Solid Edge part; units mm, degrees
sketch "Sketch1" plane through (0, 0, 0) normal (0, 0, 1) x (1, 0, 0)
  circle A0 centre (0, 0) radius 5
extrude "Protrusion1" add sketch "Sketch1" along normal blind 1.5
sketch "Sketch2" plane through (0, 0, 0) normal (0, 0, 1) x (1, 0, 0)
  line L0 (-1, 4) -> (-1, -4)
  line L1 (-1, -4) -> (1, -4)
  line L2 (1, -4) -> (1, 4)
  line L3 (1, 4) -> (-1, 4)
extrude "Protrusão_Extrudada_2" add sketch "Sketch2" along normal blind 2.3
sketch "Sketch3" plane through (0, 0, 0) normal (0, 0, 1) x (1, 0, 0)
  line L0 (-4, -1) -> (4, -1)
  line L1 (4, -1) -> (4, 1)
  line L2 (4, 1) -> (-4, 1)
  line L3 (-4, 1) -> (-4, -1)
extrude "Protrusão_Extrudada_3" add sketch "Sketch3" along normal blind 2.3
sketch "Sketch4" plane through (0, 0, 0) normal (0, 0, -1) x (-1, 0, 0)
  circle A0 centre (0, 0) radius 1
extrude "Protrusão_Extrudada_4" add sketch "Sketch4" along normal blind 6
Part model, mm, in its own coordinate system. A direction names the side the tool comes from. Give positions to 0.01 mm unless a question says otherwise; leave off trailing zeros. Write each loop counter-clockwise with the first axis right and the second up, starting at its lowest first coordinate (ties: lowest second). Pieces come first, ordered by that corner, then holes.
1) Cut at A-A on x = 0. Write the cut outline in (y, z), then the cut area to 3 significant figures.
Resolved:
outline: (-5, 0) - (-1, 0) - (-1, -6) - (1, -6) - (1, 0) - (5, 0) - (5, 1.5) - (4, 1.5) - (4, 2.3) - (-4, 2.3) - (-4, 1.5) - (-5, 1.5) - close
area: 33.4 mm2
2) Cut at C-C on y = -3.25. Write the cut outline in (x, z).
Resolved:
outline: (-3.8, 0) - (3.8, 0) - (3.8, 1.5) - (1, 1.5) - (1, 2.3) - (-1, 2.3) - (-1, 1.5) - (-3.8, 1.5) - close
3) Which spindle directions (+Z, -Z, +X, -X, +Y, -Y) get a long thin tool onto all of the face, cutting with end or side? Do faces 1 (the face through (0, 1, -3)), 2 (the face through (0, 0, -6)). Say none if no direction does.
Resolved:
face 1: -Z
face 2: -Z, +X, -X, +Y, -Y
4) Cut at D-D on y = 1.5. Write the cut outline in (x, z).
Resolved:
outline: (-4.77, 0) - (4.77, 0) - (4.77, 1.5) - (1, 1.5) - (1, 2.3) - (-1, 2.3) - (-1, 1.5) - (-4.77, 1.5) - close
5) Pin check, flat tips, straight feed: pin 1 (0.6 mm diameter, centred on x = -3, z = 2, fed in from +Y); pin 2 (0.9 mm diameter, centred on y = 0, z = 2, fed in from +X); pin 3 (0.9 mm diameter, centred on x = -2.5, z = 2, fed in from -Y); pin 4 (1.5 mm diameter, centred on x = -2, z = -3.5, fed in from +Y). Stop position of each tip, or through.
Resolved:
pin 1: stops at y = 1
pin 2: stops at x = 4
pin 3: stops at y = -1
pin 4: passes through
6) Cut at B-B on z = 1.75. Write the cut outline in (x, y).
Resolved:
outline: (-4, -1) - (-1, -1) - (-1, -4) - (1, -4) - (1, -1) - (4, -1) - (4, 1) - (1, 1) - (1, 4) - (-1, 4) - (-1, 1) - (-4, 1) - close
7) Probe L1, parallel to Z at x = -4.25, y = -2; L2, parallel to Z at x = -3.5, y = -0.5; L3, parallel to X at y = 0.75, z = -0.25. List the from-to ranges inside material, lowest first.
Resolved:
L1: z = 0 to 1.5
L2: z = 0 to 2.3
L3: x = -0.66 to 0.66
